The listing builds one solid part. Answer for the finished solid, in the listing's coordinates (mm). Face numbers are marked on the shaded views. A direction names the side the tool comes from. Give positions to 0.01 mm unless a question says otherwise; leave off trailing zeros. Order: outer loops, then holes, each group sorted by start corner. A loop starts at its lowest first (then second) coordinate and runs counter-clockwise, first axis right, second up. Notation, with made-up numbers: (10, -4.75) - (19, -4.75) arc R11 ccw to (19, 4.25) - close; hole circle Ø10 at (25.5, 45.5). An arc over 180 degrees is marked (long way). Use a Markdown table: item, result. Add a question column.
1) Find section A-A, the plane x = 0. Determine the outline of the cut face in (y, z), plus the area to 3 significant figures.
2) Find section B-B, the plane z = 85. Determine the outline of the cut face in (x, y).
3) Straight lines are drawn through the part: line 1 (Z direction, x = 0, y = 3.2); line 2 (Z direction, x = 0, y = 1.15); line 3 (X direction, y = 2.9, z = 85). For each, find the intervals that lie inside material, in ascending order.
4) Find section C-C, the plane z = 17.5. Determine the outline of the cut face in (x, y), plus the area to 3 significant figures.
5) Flat-ended cylindrical pins translate along their axes: pin 1 (14.5 mm diameter, centred on x = 0, z = -85, fed in from -Y); pin 2 (7 mm diameter, centred on x = -3, z = 27.5, fed in from +Y); pin 3 (1.8 mm diameter, centred on y = -4.5, z = 2.5, fed in from -X); pin 4 (5 mm diameter, centred on x = 1, y = -2, fed in from +Z). Find the tip coordinate at first contact, or state that the pin passes through.
6) Find section D-D, the plane x = -9.25. Determine the outline of the cut face in (y, z), plus the area to 3 significant figures.
7) For the marked faces 1 and 2, determine the directions among +Z, -Z, +X, -X, +Y, -Y from which every point of the face is accessible in a straight line to the end or side of a thin tool.
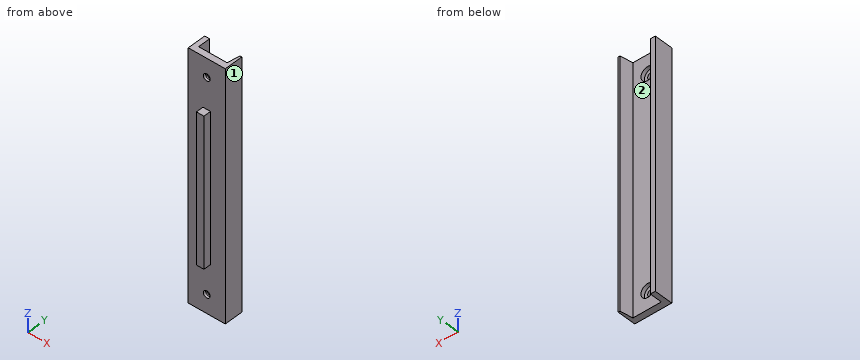
from build123d import *

# Parameters (mm, degrees)
SKETCH_1_W                   = 30
SKETCH_1_H                   = 200
EXTRUDE_1_DEPTH              = 5
SKETCH_2_W                   = 4
SKETCH_2_H                   = 200
SKETCH_2_W_2                 = 3
EXTRUDE_2_DEPTH              = 10
CUT_EXTRUDE_1_DEPTH          = 202.121853611
HOLE_WIZARD_M5_1_D           = 5.5
HOLE_WIZARD_M5_1_DEPTH       = 30
HOLE_WIZARD_M5_1_CBORE_D     = 11
HOLE_WIZARD_M5_1_CBORE_DEPTH = 3
HOLE_WIZARD_M5_1_TIP         = 1.652366702
SKETCH_7_W                   = 6.1
SKETCH_7_H                   = 120
EXTRUDE_3_DEPTH              = 6


with BuildPart() as part:
    # 스케치1 → 보스-돌출1 (new body)
    with BuildSketch(Plane(origin=(0, 0, 0), x_dir=(1, 0, 0), z_dir=(0, 1, 0))):
        Rectangle(SKETCH_1_W, SKETCH_1_H)
    extrude(amount=EXTRUDE_1_DEPTH)

    # 스케치2 → 보스-돌출2 (add)
    with BuildSketch(Plane(origin=(0, 5, 0), x_dir=(1, 0, 0), z_dir=(0, 1, 0))):
        with Locations((-13, 0)):
            Rectangle(SKETCH_2_W, SKETCH_2_H)
        with Locations((13.5, 0)):
            Rectangle(SKETCH_2_W_2, SKETCH_2_H)
    extrude(amount=EXTRUDE_2_DEPTH)

    # 스케치3 → 컷-돌출1 (cut, through all)
    with BuildSketch(Plane.XY.offset(100)):
        Polygon((12, 5), (12, 15), (13.5, 15), align=None)
    extrude(amount=-CUT_EXTRUDE_1_DEPTH, mode=Mode.SUBTRACT)

    # M5 소켓 머리 캡 나사용 카운터보어1
    with Locations(Plane(origin=(0, 5, 0), x_dir=(1, 0, 0), z_dir=(0, 1, 0))):
        with Locations((0, -85), (0, 85)):
            CounterBoreHole(HOLE_WIZARD_M5_1_D / 2, HOLE_WIZARD_M5_1_CBORE_D / 2, HOLE_WIZARD_M5_1_CBORE_DEPTH, depth=HOLE_WIZARD_M5_1_DEPTH)
            with Locations((0, 0, -(HOLE_WIZARD_M5_1_DEPTH + HOLE_WIZARD_M5_1_TIP / 2))):  # 118° drill point
                Cone(0, HOLE_WIZARD_M5_1_D / 2, HOLE_WIZARD_M5_1_TIP, mode=Mode.SUBTRACT)

    # 스케치7 → 보스-돌출3 (add)
    with BuildSketch(Plane.XZ):
        Rectangle(SKETCH_7_W, SKETCH_7_H)
    extrude(amount=EXTRUDE_3_DEPTH)


solid = part.part
The answers:
| question | item | result |
|---|---|---|
| 1 | outline | (-6, -60) - (0, -60) - (0, -82.25) - (2, -82.25) - (2, -79.5) - (5, -79.5) - (5, 79.5) - (2, 79.5) - (2, 82.25) - (0, 82.25) - (0, 60) - (-6, 60) - close; (0, -100) - (5, -100) - (5, -90.5) - (2, -90.5) - (2, -87.75) - (0, -87.75) - close; (0, 87.75) - (2, 87.75) - (2, 90.5) - (5, 90.5) - (5, 100) - (0, 100) - close |
| 1 | area | 1,630 mm2 |
| 2 | outline | (-15, 0) - (-2.75, 0) - (-2.75, 2) - (-5.5, 2) - (-5.5, 5) - (-11, 5) - (-11, 15) - (-15, 15) - close; (2.75, 0) - (15, 0) - (15, 15) - (13.5, 15) - (12, 5) - (5.5, 5) - (5.5, 2) - (2.75, 2) - close |
| 3 | line 1 | -100 to -90.5, -79.5 to 79.5, 90.5 to 100 |
| 3 | line 2 | -100 to -87.75, -82.25 to 82.25, 87.75 to 100 |
| 3 | line 3 | -15 to -5.5, 5.5 to 15 |
| 4 | outline | (-15, 0) - (-3.05, 0) - (-3.05, -6) - (3.05, -6) - (3.05, 0) - (15, 0) - (15, 15) - (13.5, 15) - (12, 5) - (-11, 5) - (-11, 15) - (-15, 15) - close |
| 4 | area | 249 mm2 |
| 5 | pin 1 | y = 0 |
| 5 | pin 2 | y = 5 |
| 5 | pin 3 | x = -3.05 |
| 5 | pin 4 | z = 100 |
| 6 | outline | (0, -100) - (5, -100) - (5, 100) - (0, 100) - close |
| 6 | area | 1,000 mm2 |
| 7 | face 1 | +Z, -Z, +X, +Y, -Y |
| 7 | face 2 | +Z, -Z, +Y |
